from build123d import *

# Parameters (mm, degrees)
SKETCH1_W           = 85
SKETCH1_H           = 50
BOSS_EXTRUDE1_DEPTH = 5.55
SKETCH2_W           = 7.75
SKETCH2_H           = 50
CUT_EXTRUDE1_DEPTH  = 3.95
SKETCH3_R           = 1.5
CUT_EXTRUDE2_DEPTH  = 2.6
SKETCH4_W           = 5.700401694
SKETCH4_H           = 17.101205084
BOSS_EXTRUDE2_DEPTH = 3
SKETCH5_W           = 8.5
SKETCH5_H           = 14.8
BOSS_EXTRUDE3_DEPTH = 7.5


with BuildPart() as part:
    # Sketch1 → Boss-Extrude1 (new body)
    with BuildSketch(Plane(origin=(0, 0, 0), x_dir=(1, 0, 0), z_dir=(0, 1, 0))):
        with Locations((42.5, 25)):
            Rectangle(SKETCH1_W, SKETCH1_H)
    extrude(amount=BOSS_EXTRUDE1_DEPTH)

    # Sketch2 → Cut-Extrude1 (cut)
    with BuildSketch(Plane(origin=(0, 5.55, 0), x_dir=(1, 0, 0), z_dir=(0, 1, 0))):
        with Locations((3.875, 25)):
            Rectangle(SKETCH2_W, SKETCH2_H)
        with Locations((81.125, 25)):
            Rectangle(SKETCH2_W, SKETCH2_H)
    extrude(amount=-CUT_EXTRUDE1_DEPTH, mode=Mode.SUBTRACT)

    # Sketch3 → Cut-Extrude2 (cut, through all)
    with BuildSketch(Plane(origin=(0, 1.6, 0), x_dir=(1, 0, 0), z_dir=(0, 1, 0))):
        with Locations((3.2, 46.8)):
            Circle(SKETCH3_R)
        with Locations((3.2, 3.2)):
            Circle(SKETCH3_R)
        with Locations((81.8, 3.2)):
            Circle(SKETCH3_R)
        with Locations((81.8, 46.8)):
            Circle(SKETCH3_R)
        with BuildLine():
            Line((0, 46.8), (0, 50))
            Line((0, 50), (3.2, 50))
            ThreePointArc((3.2, 50), (0.9372583, 49.0627417), (0, 46.8))
        make_face()
        with BuildLine():
            Line((0, 0), (3.2, 0))
            ThreePointArc((3.2, 0), (0.9372583, 0.9372583), (0, 3.2))
            Line((0, 3.2), (0, 0))
        make_face()
        with BuildLine():
            Line((85, 3.2), (85, 0))
            Line((85, 0), (81.8, 0))
            ThreePointArc((81.8, 0), (84.0627417, 0.9372583), (85, 3.2))
        make_face()
        with BuildLine():
            Line((85, 50), (81.8, 50))
            ThreePointArc((81.8, 50), (84.0627417, 49.0627417), (85, 46.8))
            Line((85, 46.8), (85, 50))
        make_face()
    extrude(amount=-CUT_EXTRUDE2_DEPTH, mode=Mode.SUBTRACT)

    # Sketch4 → Boss-Extrude2 (add)
    with BuildSketch(Plane.XZ):
        with Locations((33.858914892, -11.880027846)):
            Rectangle(SKETCH4_W, SKETCH4_H)
    extrude(amount=BOSS_EXTRUDE2_DEPTH)

    # Sketch5 → Boss-Extrude3 (add)
    with BuildSketch(Plane.XZ):
        with Locations((80.75, -25)):
            Rectangle(SKETCH5_W, SKETCH5_H)
    extrude(amount=BOSS_EXTRUDE3_DEPTH)


solid = part.part
Model file for the job. Use its own axes, mm. A direction names the side the tool comes from. Give positions to 0.01 mm unless a question says otherwise; leave off trailing zeros. Order: outer loops, then holes, each group sorted by start corner. A loop starts at its lowest first (then second) coordinate and runs counter-clockwise, first axis right, second up. Notation, with made-up numbers: (26.25, 51.25) -> (65.25, 51.25) arc R14 cw to (65.25, 64.25) -> close; hole circle Ø3 at (49.5, -25). An arc over 180 degrees is marked (long way). Use CSV: the item, a comma, the result in double quotes.
1. Band-saw the part on D-D, the plane z = -23.5. Give the cut face in (x, y), then the cut area to 3 significant figures.
Outcome:
outline,"(0, 0) -> (76.5, 0) -> (76.5, -7.5) -> (85, -7.5) -> (85, 1.6) -> (77.25, 1.6) -> (77.25, 5.55) -> (7.75, 5.55) -> (7.75, 1.6) -> (0, 1.6) -> close"
area,"474 mm²"
2. 3-axis set-ups, long thin cutter, end or side, ignore diameter. For faces 4 (the flat face through (81, -4, -17.6)), 5 (the flat face through (31.009, -1, -12)), 6 (the flat face through (77.25, 4, -25)): which of +Z, -Z, +X, -X, +Y, -Y reach the whole face in a straight line?
Outcome:
face 4,"+Z, +X, -Y"
face 5,"+Z, -Z, -X, -Y"
face 6,"+Z, -Z, +X, +Y"
3. Mould opens along X. For faces 1 (the flat face through (81, 1.6, -25)), 2 (the cylindrical face through (0.962, 0.811, -49.087)), 3 (the cylindrical face through (2.875, 0.811, -45.336)) say: +X half, -X half, draft (parallel to the pull), parting line (faces both ways), or undercut.
Outcome:
face 1,"draft"
face 2,"-X half"
face 3,"undercut"
4. Drill centre lines: line 1 along Z through (x, y) = (3.2, 1.2); line 2 along X through (y, z) = (1.05, -46.8); line 3 along Y through (x, z) = (46.5, -20). Where is each one in solid material? Low to high. Write a range as from..to.
Outcome:
line 1,"-50..-48.3, -45.3..-4.7, -1.7..0"
line 2,"0..1.7, 4.7..80.3, 83.3..85"
line 3,"0..5.55"
5. Drop flat-ended pins along their axis: pin 1 (2 mm diameter, centred on y = -2.5, z = -28, fed in from -X); pin 2 (1.5 mm diameter, centred on y = -1.5, z = -13, fed in from +X); pin 3 (1.2 mm diameter, centred on y = 2.5, z = -25, fed in from +X). Give the stop position or say it passes through.
Outcome:
pin 1,"x = 76.5"
pin 2,"x = 36.71"
pin 3,"x = 77.25"
6. Band-saw the part on A-A, the plane z = -42.5. Give the cut face in (x, y).
Outcome:
outline,"(0, 0) -> (85, 0) -> (85, 1.6) -> (77.25, 1.6) -> (77.25, 5.55) -> (7.75, 5.55) -> (7.75, 1.6) -> (0, 1.6) -> close"
7. Band-saw the part on B-B, the plane x = 79. Give the cut face in (y, z), then the cut area to 3 significant figures.
Outcome:
outline,"(-7.5, -32.4) -> (0, -32.4) -> (0, -50) -> (1.6, -50) -> (1.6, 0) -> (0, 0) -> (0, -17.6) -> (-7.5, -17.6) -> close"
area,"191 mm²"
8. Band-saw the part on C-C, the plane y = 3.5. Give the cut face in (x, z).
Outcome:
outline,"(7.75, -50) -> (77.25, -50) -> (77.25, 0) -> (7.75, 0) -> close"
